from build123d import *

# Parameters (mm, degrees)
BOSS_EXTRUDE1_DEPTH = 2
SKETCH4_R           = 1.1176
BOSS_EXTRUDE2_DEPTH = 2.54
FILLET1_R           = 2


with BuildPart() as part:
    # Sketch3 → Boss-Extrude1 (new body)
    with BuildSketch(Plane(origin=(0, 0, 0), x_dir=(1, 0, 0), z_dir=(0, 1, 0))):
        Polygon((-16, 0), (16, 0), (16, 7), (30.75, 7), (30.75, 32), (-30.75, 32), (-30.75, 7), (-16, 7), align=None)
    extrude(amount=BOSS_EXTRUDE1_DEPTH)

    # Sketch4 → Boss-Extrude2 (add)
    with BuildSketch(Plane(origin=(0, 2, 0), x_dir=(1, 0, 0), z_dir=(0, 1, 0))):
        with Locations(Location((-28.44, 9.31, 0), (0, 0, 270))):
            Circle(SKETCH4_R)
        with Locations(Location((-28.44, 29.63, 0), (0, 0, 270))):
            Circle(SKETCH4_R)
        with Locations(Location((28.44076, 29.63, 0), (0, 0, 270))):
            Circle(SKETCH4_R)
        with Locations(Location((28.44076, 9.31, 0), (0, 0, 270))):
            Circle(SKETCH4_R)
    extrude(amount=BOSS_EXTRUDE2_DEPTH)

    # Fillet1
    fillet1_edges = [part.edges().sort_by_distance(p)[0] for p in [
        (-30.75, 1, -7),
        (-30.75, 1, -32),
        (30.75, 1, -32),
        (30.75, 1, -7),
    ]]
    fillet(fillet1_edges, radius=FILLET1_R)


solid = part.part
Could you check a few things on this model? Use its own coordinates, in mm. A direction names the side the tool comes from. Give positions to 0.01 mm unless a question says otherwise; leave off trailing zeros. Order: outer loops, then holes, each group sorted by start corner. A loop starts at its lowest first (then second) coordinate and runs counter-clockwise, first axis right, second up. Notation, with made-up numbers: M 27,50 L 39,50 A20 ccw 39,64 Z; hole C 55.25,51.5 d11. An arc over 180 degrees is marked long. One line per question, with ' | ' between items.
1. For faces 4 (the face through (30.18, 1.01, -31.4)), 5 (the face through (0, 1, 0)), 6 (the face through (-16, 1, -4)), 7 (the face through (-28.87, 3.25, -28.6)), 8 (the face through (22, 1, -7)), which set-ups out of +Z, -Z, +X, -X, +Y, -Y let a thin tool reach every point of the face, with its end or its side?
Results:
face 4: -Z, +X, +Y, -Y | face 5: +Z, +X, -X, +Y, -Y | face 6: +Z, -X, +Y, -Y | face 7: +Y | face 8: +Z, +X, +Y, -Y
2. We'd pull the mould along Z, two halves only. Please class faces 1 (the face through (-30.15, 1.01, -7.57)), 2 (the face through (30.75, 1, -19)), 3 (the face through (-29.12, 3.252, -10.197)): +Z half, -Z half, draft (parallel to the pull), parting line (faces both ways), or undercut.
Results:
face 1: +Z half | face 2: draft | face 3: undercut
3. I want a section at B-B (z = -2.5). List the corners of the cut face in (x, y) for me, and give its area (3 significant figures).
Results:
outline: M -16,0 L 16,0 L 16,2 L -16,2 Z | area: 64.0 mm²
4. If I drill on line 1 (Z direction, x = -24, y = 1.2); line 2 (Y direction, x = 0.5, z = -14); line 3 (X direction, y = 3.75, z = -10), over which ranges is the centre line in solid material (lowest first)?
Results:
line 1: -32 to -7 | line 2: 0 to 2 | line 3: -29.32 to -27.56, 27.56 to 29.32
5. I want a section at C-C (x = -24.5). List the corners of the cut face in (y, z) for me.
Results:
outline: M 0,-32 L 2,-32 L 2,-7 L 0,-7 Z
6. I'm going to push flat-ended pins straight in: pin 1 (0.6 mm diameter, centred on y = 1, z = -3, fed in from +X); pin 2 (1 mm diameter, centred on x = -24, y = 1, fed in from +Z); pin 3 (12 mm diameter, centred on x = 19, z = -4, fed in from +Y). Where does each tip first touch, or does it pass through?
Results:
pin 1: x = 16 | pin 2: z = -7 | pin 3: y = 2
7. I want a section at A-A (y = 0.7). List the corners of the cut face in (x, z) for me, and give its area (3 significant figures).
Results:
outline: M -30.75,-30 A2 ccw -28.75,-32 L 28.75,-32 A2 ccw 30.75,-30 L 30.75,-9 A2 ccw 28.75,-7 L 16,-7 L 16,0 L -16,0 L -16,-7 L -28.75,-7 A2 ccw -30.75,-9 Z | area: 1,760 mm²
